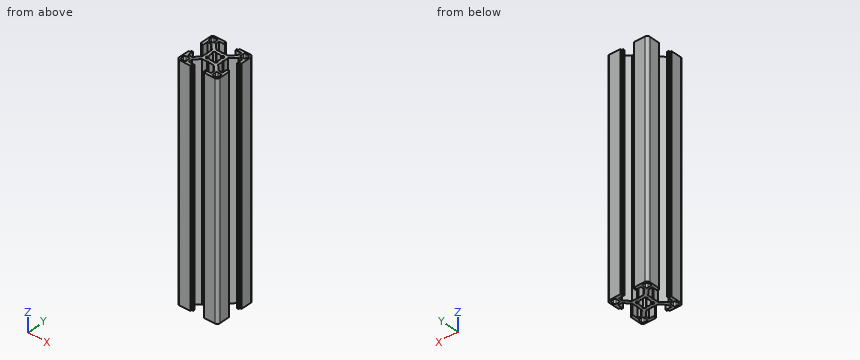
```python
from build123d import *

# Parameters (mm, degrees)
SKETCH1_R                = 3.65
SKETCH1_W                = 4
SKETCH1_H                = 4
BOSS_EXTRUDE1_DEPTH      = 168
FILLET1_R                = 1
CIRPATTERN1_COUNT        = 4
FILLET1_OF_CIRPATTERN1_R = 1
CUT_EXTRUDE1_DEPTH       = 170.3339895
CUT_EXTRUDE2_DEPTH       = 170.3339895
CIRPATTERN2_COUNT        = 4


with BuildPart() as part:
    # Sketch1 → Boss-Extrude1 (new body)
    with BuildSketch(Plane.XY):
        with BuildLine():
            Line((5.1, 15), (13, 15))
            ThreePointArc((13, 15), (14.414213562, 14.414213562), (15, 13))
            Line((15, 13), (15, 5.1))
            Line((15, 5.1), (13.9, 5.1))
            Line((13.9, 5.1), (13.9, 4))
            Line((13.9, 4), (12.8, 4))
            Line((12.8, 4), (12.8, 8.25))
            Line((12.8, 8.25), (10.017766953, 8.25))
            Line((10.017766953, 8.25), (6, 4.232233047))
            Line((6, 4.232233047), (6, -6))
            Line((6, -6), (-6, -6))
            Line((-6, -6), (-6, 6))
            Line((-6, 6), (4.232233047, 6))
            Line((4.232233047, 6), (8.25, 10.017766953))
            Line((8.25, 10.017766953), (8.25, 12.8))
            Line((8.25, 12.8), (4, 12.8))
            Line((4, 12.8), (4, 13.9))
            Line((4, 13.9), (5.1, 13.9))
            Line((5.1, 13.9), (5.1, 15))
        make_face()
        with Locations(Location((0, 0, 0), (0, 0, 180))):
            Circle(SKETCH1_R, mode=Mode.SUBTRACT)
        with Locations((11.75, 11.75)):
            Rectangle(SKETCH1_W, SKETCH1_H, mode=Mode.SUBTRACT)
    boss_extrude1 = extrude(amount=BOSS_EXTRUDE1_DEPTH)

    # Fillet1
    fillet1_edges = [part.edges().sort_by_distance(p)[0] for p in [
        (9.75, 13.75, 84),
        (9.75, 9.75, 84),
        (13.75, 9.75, 84),
        (13.75, 13.75, 84),
    ]]
    fillet(fillet1_edges, radius=FILLET1_R)

    # CirPattern1: Boss-Extrude1 ×4 about axis
    cirpattern1_axis = Axis((0, 0, 0), (0, 0, 1))
    for i in range(1, CIRPATTERN1_COUNT):
        add(boss_extrude1.rotate(cirpattern1_axis, i * 360 / CIRPATTERN1_COUNT))

    # Fillet1 of CirPattern1
    fillet1_of_cirpattern1_edges = [part.edges().sort_by_distance(p)[0] for p in [
        (-13.75, 9.75, 84),
        (-9.75, 9.75, 84),
        (-9.75, 13.75, 84),
        (-13.75, 13.75, 84),
        (-9.75, -13.75, 84),
        (-9.75, -9.75, 84),
        (-13.75, -9.75, 84),
        (-13.75, -13.75, 84),
        (13.75, -9.75, 84),
        (9.75, -9.75, 84),
        (9.75, -13.75, 84),
        (13.75, -13.75, 84),
    ]]
    fillet(fillet1_of_cirpattern1_edges, radius=FILLET1_OF_CIRPATTERN1_R)

    # Sketch2 → Cut-Extrude1 (cut, through all)
    with BuildSketch(Plane(origin=(0, 0, 0), x_dir=(-1, 0, 0), z_dir=(0, 0, -1))):
        Polygon((0, 5.5), (-0.5, 6), (0.5, 6), align=None)
    cut_extrude1 = extrude(amount=-CUT_EXTRUDE1_DEPTH, mode=Mode.SUBTRACT)

    # Sketch3 → Cut-Extrude2 (cut, through all)
    with BuildSketch(Plane(origin=(0, 0, 0), x_dir=(-1, 0, 0), z_dir=(0, 0, -1))):
        with BuildLine():
            Line((-1.775079755, 3.189293317), (-2.828427125, 4.242640687))
            Line((-2.828427125, 4.242640687), (-4.242640687, 2.828427125))
            Line((-4.242640687, 2.828427125), (-3.189293317, 1.775079755))
            ThreePointArc((-3.189293317, 1.775079755), (-2.580939751, 2.580939751), (-1.775079755, 3.189293317))
        make_face()
    cut_extrude2 = extrude(amount=-CUT_EXTRUDE2_DEPTH, mode=Mode.SUBTRACT)

    # CirPattern2: Cut-Extrude1, Cut-Extrude2 ×4 about axis
    cirpattern2_axis = Axis((0, 0, 0), (0, 0, 1))
    add([cut_extrude1.rotate(cirpattern2_axis, i * 360 / CIRPATTERN2_COUNT) for i in range(1, CIRPATTERN2_COUNT)], mode=Mode.SUBTRACT)
    add([cut_extrude2.rotate(cirpattern2_axis, i * 360 / CIRPATTERN2_COUNT) for i in range(1, CIRPATTERN2_COUNT)], mode=Mode.SUBTRACT)


solid = part.part
```
Build history of the part. All positions in model axes, mm. Round coordinates to 2 decimals unless told otherwise and drop trailing zeros.
1) Pin check, flat tips, straight feed: pin 1 (0.5 mm diameter, centred on x = 13.5, z = 107, fed in from +Y); pin 2 (0.9 mm diameter, centred on x = -4.5, z = 123, fed in from -Y); pin 3 (3 mm diameter, centred on x = -1.5, z = 102.5, fed in from +Y); pin 4 (1.5 mm diameter, centred on x = -7.5, y = -4.5, fed in from -Z). Stop position of each tip, or through.
2) Band-saw the part on A-A, the plane z = 90. Give the number of separate pieces and of enclosed holes in the cut face, and give its area (3 significant figures).
3) Drill centre lines: probe 1 along X at (y, z) = (11.5, 72.5); probe 2 along X at (y, z) = (-10, 154.5). Where is each one in solid material? Low to high.
Ans:
1. pin 1: stops at y = 14.98
1. pin 2: stops at y = -13.9
1. pin 3: stops at y = 6
1. pin 4: passes through
2. separate pieces: 1
2. enclosed holes: 5
2. area: 318 mm2
3. probe 1: x = -15 to -13.75, -9.75 to -8.25, 8.25 to 9.75, 13.75 to 15
3. probe 2: x = -15 to -13.41, -10.09 to -8.23, 8.23 to 10.09, 13.41 to 15
